Check sheet for the modelled part. Datum: model origin and axes. Units: mm. Round coordinates to 2 decimals unless told otherwise and drop trailing zeros. Loops run counter-clockwise (first coordinate to the right, second up) from the corner with the lowest first, then second, coordinate; pieces in that order, holes last. Notation, with made-up numbers: (-7, -11) - (49, -11) arc R21 cw to (49, 19) - close; hole circle Ø1 at (84.5, 25). An arc over 180 degrees is marked (long way). Return JSON: item names as keys, results as strings.
from build123d import *

# Parameters (mm, degrees)
EXTRUDE_1_DEPTH          = 63
SKETCH_2_W               = 37.314872722
SKETCH_2_H               = 5
CUT_EXTRUDE_1_DEPTH      = 50
PATTERN_LINEAR_1_COUNT   = 6
PATTERN_LINEAR_1_PITCH   = 11
MIRROR_1_COPY_1_SKETCH_W = 37.314872722
MIRROR_1_COPY_1_SKETCH_H = 5
MIRROR_1_COPY_1_DEPTH    = 50
MIRROR_1_COPY_2_SKETCH_W = 37.314872722
MIRROR_1_COPY_2_SKETCH_H = 5
MIRROR_1_COPY_2_DEPTH    = 50
MIRROR_1_COPY_3_SKETCH_W = 37.314872722
MIRROR_1_COPY_3_SKETCH_H = 5
MIRROR_1_COPY_3_DEPTH    = 50
MIRROR_1_COPY_4_SKETCH_W = 37.314872722
MIRROR_1_COPY_4_SKETCH_H = 5
MIRROR_1_COPY_4_DEPTH    = 50
MIRROR_1_COPY_5_SKETCH_W = 37.314872722
MIRROR_1_COPY_5_SKETCH_H = 5
MIRROR_1_COPY_5_DEPTH    = 50
MIRROR_1_COPY_6_SKETCH_W = 37.314872722
MIRROR_1_COPY_6_SKETCH_H = 5
MIRROR_1_COPY_6_DEPTH    = 50
EXTRUDE_START            = 63
SKETCH_3_R               = 2.5
EXTRUDE_2_DEPTH          = 20
SKETCH_4_R               = 2.5
EXTRUDE_3_DEPTH          = 20


with BuildPart() as part:
    # 草图1 → 凸台-拉伸1 (new, symmetric)
    with BuildSketch(Plane.XY):
        with BuildLine():
            Line((2.857513076, 0), (30, 0))
            Line((30, 0), (30, 2))
            Line((30, 2), (11.342563639, 2))
            Line((11.342563639, 2), (2.814101031, 0.496201938))
            ThreePointArc((2.814101031, 0.496201938), (2.608464401, 0.228211064), (2.857513076, 0))
        make_face()
    extrude(amount=EXTRUDE_1_DEPTH, both=True)

    # 草图2 → 切除-拉伸1 (cut, symmetric)
    with BuildSketch(Plane(origin=(0, 2, 0), x_dir=(1, 0, 0), z_dir=(0, 1, 0))):
        with Locations((30, 0)):
            Rectangle(SKETCH_2_W, SKETCH_2_H)
    cut_extrude_1 = extrude(amount=CUT_EXTRUDE_1_DEPTH, both=True, mode=Mode.SUBTRACT)

    # 阵列(线性)1: 切除-拉伸1 ×6
    with Locations(*[(0, 0, -i * PATTERN_LINEAR_1_PITCH) for i in range(1, PATTERN_LINEAR_1_COUNT)]):
        add(cut_extrude_1, mode=Mode.SUBTRACT)

    # 镜向1 copy 1 sketch → 镜向1 copy 1 (cut, symmetric)
    with BuildSketch(Plane(origin=(0, 2, 11), x_dir=(1, 0, 0), z_dir=(0, 1, 0))):
        with Locations((30, 0)):
            Rectangle(MIRROR_1_COPY_1_SKETCH_W, MIRROR_1_COPY_1_SKETCH_H)
    extrude(amount=MIRROR_1_COPY_1_DEPTH, both=True, mode=Mode.SUBTRACT)

    # 镜向1 copy 2 sketch → 镜向1 copy 2 (cut, symmetric)
    with BuildSketch(Plane(origin=(0, 2, 22), x_dir=(1, 0, 0), z_dir=(0, 1, 0))):
        with Locations((30, 0)):
            Rectangle(MIRROR_1_COPY_2_SKETCH_W, MIRROR_1_COPY_2_SKETCH_H)
    extrude(amount=MIRROR_1_COPY_2_DEPTH, both=True, mode=Mode.SUBTRACT)

    # 镜向1 copy 3 sketch → 镜向1 copy 3 (cut, symmetric)
    with BuildSketch(Plane(origin=(0, 2, 33), x_dir=(1, 0, 0), z_dir=(0, 1, 0))):
        with Locations((30, 0)):
            Rectangle(MIRROR_1_COPY_3_SKETCH_W, MIRROR_1_COPY_3_SKETCH_H)
    extrude(amount=MIRROR_1_COPY_3_DEPTH, both=True, mode=Mode.SUBTRACT)

    # 镜向1 copy 4 sketch → 镜向1 copy 4 (cut, symmetric)
    with BuildSketch(Plane(origin=(0, 2, 44), x_dir=(1, 0, 0), z_dir=(0, 1, 0))):
        with Locations((30, 0)):
            Rectangle(MIRROR_1_COPY_4_SKETCH_W, MIRROR_1_COPY_4_SKETCH_H)
    extrude(amount=MIRROR_1_COPY_4_DEPTH, both=True, mode=Mode.SUBTRACT)

    # 镜向1 copy 5 sketch → 镜向1 copy 5 (cut, symmetric)
    with BuildSketch(Plane(origin=(0, 2, 55), x_dir=(1, 0, 0), z_dir=(0, 1, 0))):
        with Locations((30, 0)):
            Rectangle(MIRROR_1_COPY_5_SKETCH_W, MIRROR_1_COPY_5_SKETCH_H)
    extrude(amount=MIRROR_1_COPY_5_DEPTH, both=True, mode=Mode.SUBTRACT)

    # 镜向1 copy 6 sketch → 镜向1 copy 6 (cut, symmetric)
    with BuildSketch(Plane(origin=(0, 2, 0), x_dir=(1, 0, 0), z_dir=(0, 1, 0))):
        with Locations((30, 0)):
            Rectangle(MIRROR_1_COPY_6_SKETCH_W, MIRROR_1_COPY_6_SKETCH_H)
    extrude(amount=MIRROR_1_COPY_6_DEPTH, both=True, mode=Mode.SUBTRACT)

    # 草图3 → 凸台-拉伸2 (add)
    with BuildSketch(Plane.XY.offset(EXTRUDE_START)):
        with Locations(Location((5.155322669, 0.262603589, 0), (0, 0, 176.797698594))):
            Circle(SKETCH_3_R)
    extrude_2 = extrude(amount=EXTRUDE_2_DEPTH)

    # 镜向2: 凸台-拉伸2 across plane
    add(extrude_2.mirror(Plane.XY))

    # 草图4 → 凸台-拉伸3 (add, through all)
    with BuildSketch(Plane.XY.offset(63)):
        with Locations(Location((26.90226766, 0.725038627, 0), (0, 0, 196.858881031))):
            Circle(SKETCH_4_R)
    extrude(amount=EXTRUDE_3_DEPTH)


solid = part.part
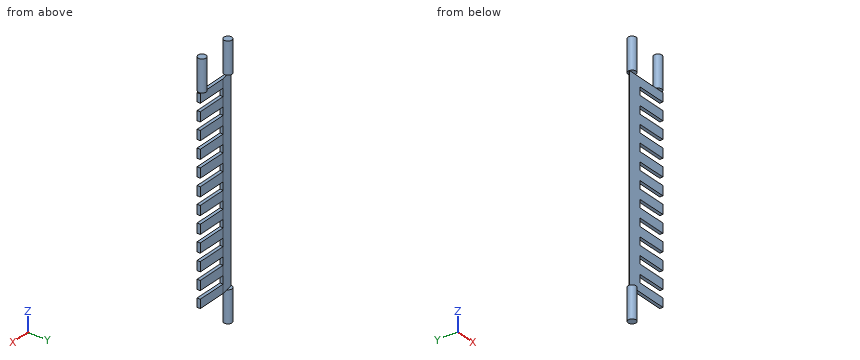
Q1. Depth check by flat-ended pin: P1, Ø10, axis at x = 23.5, z = -56.5, coming from the -Y side; P2, Ø1.6, axis at x = 23.5, y = 1.5, coming from the +Z side; P3, Ø5, axis at x = 18.5, z = -39.5, coming from the +Y side. Enter the tip coordinate at first touch or a pass-through.
Answer key:
{"P1": "stops at y = 0", "P2": "stops at z = 63", "P3": "stops at y = 2"}
Q2. Sectioned sample at A-A (x = 17). State how many separate pieces and enclosed holes the cut face has, plus the area to 3 significant figures.
Answer key:
{"separate pieces": "12", "enclosed holes": "0", "area": "142 mm²"}
Q3. Sectioned sample at D-D (z = -61). Enter the section's corners in (x, y).
Answer key:
{"outline": "(2.81, 0.5) arc R0.25 ccw to (2.86, 0) - (30, 0) - (30, 2) - (11.34, 2) - close"}
Q4. Sectioned sample at C-C (x = 4.75). Enter the section's corners in (y, z).
Answer key:
{"outline": "(-2.2, -83) - (2.73, -83) - (2.73, -63) - (0.84, -63) - (0.84, 63) - (2.73, 63) - (2.73, 83) - (-2.2, 83) - (-2.2, 63) - (0, 63) - (0, -63) - (-2.2, -63) - close"}
Q5. Sectioned sample at B-B (z = 11.5). Enter the section's corners in (x, y), plus the area to 3 significant figures.
Answer key:
{"outline": "(2.81, 0.5) arc R0.25 ccw to (2.86, 0) - (11.34, 0) - (11.34, 2) - close", "area": "10.7 mm²"}
Q6. Scan lines: probe 1 along Z at (x, y) = (26.75, 2.45); probe 2 along Y at (x, z) = (21.75, 14); probe 3 along X at (y, z) = (0.35, 25.5). Record each from-to range of solid material in increasing order. Write a range as [from, to].
Answer key:
{"probe 1": "z = [63, 83]", "probe 2": "y = [0, 2]", "probe 3": "x = [2.63, 30]"}
